Here's how the part is built. I have some questions about the finished solid (model axes, mm). A direction names the side the tool comes from. Give positions to 0.01 mm unless a question says otherwise; leave off trailing zeros. Loops run counter-clockwise (first coordinate to the right, second up) from the corner with the lowest first, then second, coordinate; pieces in that order, holes last. Notation, with made-up numbers: M 79,41 L 94,41 A21 ccw 94,59 Z; hole C 15.25,-33 d8. An arc over 180 degrees is marked long. Answer as CSV lines item,"result". Start each with the question number.
Item 1: If I drill on line 1 along Y through (x, z) = (0.25, 0.5); line 2 along X through (y, z) = (8, -17); line 3 along X through (y, z) = (-13.4, 17), over which ranges is the centre line in solid material (lowest first)? Write a range as from..to.
Item 2: For faces 4 (the conical face through (0.999, 20.573, -18.303)), 5 (the flat face through (-8, -17.24, 5.69)), 6 (the cylindrical face through (-0.07, 14.64, -18.5)), which set-ups out of +Z, -Z, +X, -X, +Y, -Y let a thin tool reach every point of the face, with its end or its side?
Item 3: Will these pins go through, and if not, where does the flat tip stop? P1, Ø4.5, axis at x = -0.5, z = -17.5, coming from the -Y side; P2, Ø1.2, axis at x = 0, z = 17, coming from the +Y side; P3, Ø6.5, axis at x = 0.5, z = -17.5, coming from the +Y side.
Item 4: I want a section at B-B on y = 23. List the corners of the cut face in (x, z) for me.
Item 5: I want a section at C-C on x = 3.75. List the corners of the cut face in (y, z) for me, plus the area to 3 significant figures.
Item 6: If we mould it in two halves opening along Y, with no side actions, what happens to faces 1 (the conical face through (0.999, -20.573, 18.303)), 2 (the cylindrical face through (0, 26, 0)), 3 (the flat face through (8, -8, 0))? For each: released by +Y, released by -Y, zero draft, split by the parting line, or undercut.
Item 7: I want a section at A-A on z = 0. List the corners of the cut face in (x, y) for me, plus the area to 3 significant figures.
from build123d import *

# Parameters (mm, degrees)
SKETCH2_R           = 2
BODY_DEPTH          = 8.5
SKETCH10_R          = 7.5
CUT_EXTRUDE2_DEPTH  = 10
SKETCH3_R           = 8.5
O_RING_SEAT_DEPTH   = 0.5
SKETCH8_R           = 18
CAVITY_DEPTH        = 7
SKETCH5_R           = 1
OUTLET_DEPTH        = 38.739236876
BOSS_EXTRUDE2_REACH = 50.576
SKETCH6_R           = 3
SKETCH6_R_2         = 1
INLET_COUNT         = 2
CUT_EXTRUDE3_REACH  = 42.509
SKETCH11_R          = 18
SKETCH12_R          = 19.5
CUT_EXTRUDE4_DEPTH  = 0.5


with BuildPart() as part:
    # Sketch2 → Body (new, symmetric)
    with BuildSketch(Plane(origin=(0, 0, 0), x_dir=(0, 0, -1), z_dir=(1, 0, 0))):
        with BuildLine():
            ThreePointArc((-14.142135624, 14.142135624), (-26, 0), (-14.142135624, -14.142135624))
            ThreePointArc((-14.142135624, -14.142135624), (0, -26), (14.142135624, -14.142135624))
            ThreePointArc((14.142135624, -14.142135624), (26, 0), (14.142135624, 14.142135624))
            ThreePointArc((14.142135624, 14.142135624), (0, 26), (-14.142135624, 14.142135624))
        make_face()
        with Locations((0, 23)):
            Circle(SKETCH2_R, mode=Mode.SUBTRACT)
        with Locations((23, 0)):
            Circle(SKETCH2_R, mode=Mode.SUBTRACT)
        with Locations((0, -23)):
            Circle(SKETCH2_R, mode=Mode.SUBTRACT)
        with Locations((-23, 0)):
            Circle(SKETCH2_R, mode=Mode.SUBTRACT)
    extrude(amount=BODY_DEPTH, both=True)

    # Sketch10 → Cut-Extrude2 (cut)
    with BuildSketch(Plane(origin=(8.5, 0, 0), x_dir=(0, 0, -1), z_dir=(1, 0, 0))):
        Circle(SKETCH10_R)
    extrude(amount=-CUT_EXTRUDE2_DEPTH, mode=Mode.SUBTRACT)

    # Sketch3 → O-Ring Seat (cut)
    with BuildSketch(Plane(origin=(8.5, 0, 0), x_dir=(0, 0, -1), z_dir=(1, 0, 0))):
        Circle(SKETCH3_R)
    extrude(amount=-O_RING_SEAT_DEPTH, mode=Mode.SUBTRACT)

    # Sketch8 → Cavity (cut, symmetric)
    with BuildSketch(Plane.ZY):
        Circle(SKETCH8_R)
    extrude(amount=CAVITY_DEPTH, both=True, mode=Mode.SUBTRACT)

    # Sketch5 → Outlet (cut, through all)
    with BuildSketch(Plane(origin=(0, 0, 0), x_dir=(1, 0, 0), z_dir=(0, 1, 0))):
        with Locations(Location((0, 17, 0), (0, 0, 90))):
            Circle(SKETCH5_R)
    outlet = extrude(amount=OUTLET_DEPTH, mode=Mode.SUBTRACT)

    # Sketch6 → Boss-Extrude2 (add, up to next)
    with BuildSketch(Plane(origin=(0, 14.142135624, 0), x_dir=(1, 0, 0), z_dir=(0, 1, 0)), mode=Mode.PRIVATE) as boss_extrude2_sk1:
        with Locations((0, 17)):
            Circle(SKETCH6_R)
        with Locations(Location((0, 17, 0), (0, 0, 90))):
            Circle(SKETCH6_R_2, mode=Mode.SUBTRACT)
    boss_extrude2_tool1 = extrude(boss_extrude2_sk1.sketch, amount=-BOSS_EXTRUDE2_REACH, mode=Mode.PRIVATE) - part.part
    boss_extrude2 = boss_extrude2_tool1.solids().sort_by_distance((-2.915147, 14.142136, -17))[0]
    add(boss_extrude2)

    # Sketch9 → Revolve1 (revolve)
    with BuildSketch(Plane(origin=(0, 0, 0), x_dir=(0, 0, -1), z_dir=(1, 0, 0)), mode=Mode.PRIVATE) as revolve1_sk:
        Polygon((18, 14.142135624), (18, 21.142135624), (18.5, 21.142135624), (19, 19.142135624), (18.5, 19.142135624), (19, 17.142135624), (18.5, 17.142135624), (19, 15.142135624), (18.5, 15.142135624), (18.5, 14.142135624), align=None)
    revolve1 = revolve(revolve1_sk.sketch.rotate(Axis((0, 14.142135624, -17), (0, -1, 0)), 180), axis=Axis((0, 14.142135624, -17), (0, -1, 0)))

    # Inlet: Outlet, Boss-Extrude2, Revolve1 ×2 about axis
    inlet_axis = Axis((8, 0, 0), (1, 0, 0))
    add([outlet.rotate(inlet_axis, i * 360 / INLET_COUNT) for i in range(1, INLET_COUNT)], mode=Mode.SUBTRACT)
    add([boss_extrude2.rotate(inlet_axis, i * 360 / INLET_COUNT) for i in range(1, INLET_COUNT)])
    add([revolve1.rotate(inlet_axis, i * 360 / INLET_COUNT) for i in range(1, INLET_COUNT)])

    # Sketch11 → Cut-Extrude3 (cut, up to next)
    with BuildSketch(Plane.ZY.offset(8.5), mode=Mode.PRIVATE) as cut_extrude3_sk1:
        Circle(SKETCH11_R)
    cut_extrude3_tool1 = extrude(cut_extrude3_sk1.sketch, amount=-CUT_EXTRUDE3_REACH, mode=Mode.PRIVATE) & part.part
    add(cut_extrude3_tool1.solids().sort_by_distance((-8.5, 0, 0))[0], mode=Mode.SUBTRACT)

    # Sketch12 → Cut-Extrude4 (cut)
    with BuildSketch(Plane.ZY.offset(8.5)):
        Circle(SKETCH12_R)
    extrude(amount=-CUT_EXTRUDE4_DEPTH, mode=Mode.SUBTRACT)


solid = part.part
Result:
1,line 1,"-25.99..-24.94, -21.06..-17.99, 17.99..21.06, 24.94..25.99"
1,line 2,"-8..-1, 1..8.5"
1,line 3,"-3..-1, 1..3"
2,face 4,"+Y"
2,face 5,"-X"
2,face 6,"none"
3,P1,"y = -13.9"
3,P2,"y = 13.55"
3,P3,"y = 21.14"
4,outline,"M -8.5,-8.78 L 8.5,-8.78 L 8.5,-2 L -8.5,-2 Z; M -8.5,2 L 8.5,2 L 8.5,8.78 L -8.5,8.78 Z"
5,outline,"M -14.14,-14.14 A14.36 ccw 14.14,-14.14 A14.36 ccw 14.14,14.14 A14.36 ccw -14.14,14.14 A14.36 ccw Z; hole C -23,0 d4; hole C 0,0 d36; hole C 0,-23 d4; hole C 0,23 d4; hole C 23,0 d4"
5,area,"742 mm^2"
6,face 1,"released by -Y"
6,face 2,"released by +Y"
6,face 3,"undercut"
7,outline,"M -8.5,-26 L 8.5,-26 L 8.5,-25 L -8.5,-25 Z; M -8.5,-21 L 8.5,-21 L 8.5,-8.5 L 8,-8.5 L 8,-7.5 L 7,-7.5 L 7,-18 L -8,-18 L -8,-19.5 L -8.5,-19.5 Z; M -8.5,19.5 L -8,19.5 L -8,18 L 7,18 L 7,7.5 L 8,7.5 L 8,8.5 L 8.5,8.5 L 8.5,21 L -8.5,21 Z; M -8.5,25 L 8.5,25 L 8.5,26 L -8.5,26 Z"
7,area,"165 mm^2"
